```python
from build123d import *

# Parameters (mm, degrees)
F0_R     = 11.5
F1_DEPTH = 20


with BuildPart() as f1:
    # F0 (on Front) → F1 (new body)
    with BuildSketch(Plane.XZ):
        with BuildLine():
            ThreePointArc((12.0363, 15.97271), (3.042468, 19.76723), (-6.676137, 18.85283))
            Line((-6.676137, 18.85283), (-66.2225, -2.233643))
            ThreePointArc((-66.2225, -2.233643), (-69.85617, -3.148044), (-73.596627, -3.36863))
            Line((-73.596627, -3.36863), (-87.016434, -2.9))
            ThreePointArc((-87.016434, -2.9), (-89.245869, -3.892608), (-90, -6.213585))
            Line((-90, -6.213585), (-88.550989, -20))
            Line((-88.550989, -20), (-4.2, -20))
            ThreePointArc((-4.2, -20), (-2.057365, -20.115103), (0.060608, -20.459089))
            Line((0.060608, -20.459089), (39.351254, -29.025835))
            ThreePointArc((39.351254, -29.025835), (43.011955, -30.642935), (45.746406, -33.56501))
            ThreePointArc((45.746406, -33.56501), (50.366632, -37.660248), (56.526688, -38.073967))
            ThreePointArc((56.526688, -38.073967), (57.118662, -37.674275), (57.292966, -36.981596))
            Line((57.292966, -36.981596), (55.328237, -20.504889))
            ThreePointArc((55.328237, -20.504889), (54.06755, -16.704051), (51.416732, -13.702574))
            Line((51.416732, -13.702574), (12.0363, 15.97271))
        make_face()
        Circle(F0_R, mode=Mode.SUBTRACT)
    extrude(amount=F1_DEPTH)


solid = f1.part
```
Input: part model. Units: mm. Frame: model coordinates. A direction names the side the tool comes from. Give positions to 0.01 mm unless a question says otherwise; leave off trailing zeros. Order: outer loops, then holes, each group sorted by start corner. A loop starts at its lowest first (then second) coordinate and runs counter-clockwise, first axis right, second up.
1. Mould query, pull axis Z, two halves, no side actions, for faces 1 (the cylindrical face through (42.966, -9.86, -30.61)), 2 (the flat face through (32, -9.86, 0.93)), 3 (the flat face through (-17, 0, -9)), 4 (the cylindrical face through (-1.5, -9.9, 11.4)). Classes: released by +Z, released by -Z, zero draft, split by the parting line, or undercut.
Derived:
face 1: released by -Z
face 2: released by +Z
face 3: zero draft
face 4: undercut
2. Section D-D on x = -16. Return the cut outline in (y, z).
Derived:
outline: (-20, -20) - (0, -20) - (0, 15.55) - (-20, 15.55) - close
3. Reachability of faces 5 (the cylindrical face through (-69.8, -9.86, -3.14)), 6 (the flat face through (56.324, -9.86, -28.859)), 7 (the flat face through (-47, -10, -20)) from +Z, -Z, +X, -X, +Y, -Y: full face, straight path, thin tool, end or side. Return the list, or none.
Derived:
face 5: +Z, +Y, -Y
face 6: +Z, +X, +Y, -Y
face 7: -Z, -X, +Y, -Y
4. Section C-C on x = 8. Return the cut outline in (y, z), and give its area (3 significant figures).
Derived:
outline: (-20, -22.19) - (0, -22.19) - (0, -8.26) - (-20, -8.26) - close; (-20, 8.26) - (0, 8.26) - (0, 18.33) - (-20, 18.33) - close
area: 480 mm2
5. Section B-B on z = -9.5. Return the cut outline in (x, y), and give its area (3 significant figures).
Derived:
outline: (-89.65, -20) - (-6.48, -20) - (-6.48, 0) - (-89.65, 0) - close; (6.48, -20) - (45.84, -20) - (45.84, 0) - (6.48, 0) - close
area: 2,450 mm2
6. Section A-A on y = -18.25. Return the cut outline in (x, z).
Derived:
outline: (-90, -6.21) - (-88.55, -20) - (-4.2, -20) arc R20 cw to (0.06, -20.46) - (39.35, -29.03) arc R10.01 cw to (45.75, -33.57) arc R9.55 ccw to (56.53, -38.07) arc R1 ccw to (57.29, -36.98) - (55.33, -20.5) arc R10 ccw to (51.42, -13.7) - (12.04, 15.97) arc R20 ccw to (-6.68, 18.85) - (-66.22, -2.23) arc R20 cw to (-73.6, -3.37) - (-87.02, -2.9) arc R3 ccw to start; hole circle Ø23 at (0, 0)
7. Material intervals for L1, parallel to Z at x = 0, y = -8; L2, parallel to X at y = -16.5, z = -8; L3, parallel to Z at x = -26.5, y = -12.5, sorted ascending.
Derived:
L1: z = -20.45 to -11.5, 11.5 to 20
L2: x = -89.81 to -8.26, 8.26 to 43.85
L3: z = -20 to 11.83
8. Pin query (flat end, axial travel): pin 1 (3 mm diameter, centred on x = 35, y = -13.5, fed in from +Z); pin 2 (1 mm diameter, centred on x = -37, y = -2.5, fed in from -Z); pin 3 (1 mm diameter, centred on x = 35.5, y = -2, fed in from +Z). Return the tip coordinate at first contact, or that it passes through.
Derived:
pin 1: stops at z = -0.2
pin 2: stops at z = -20
pin 3: stops at z = -1.33
